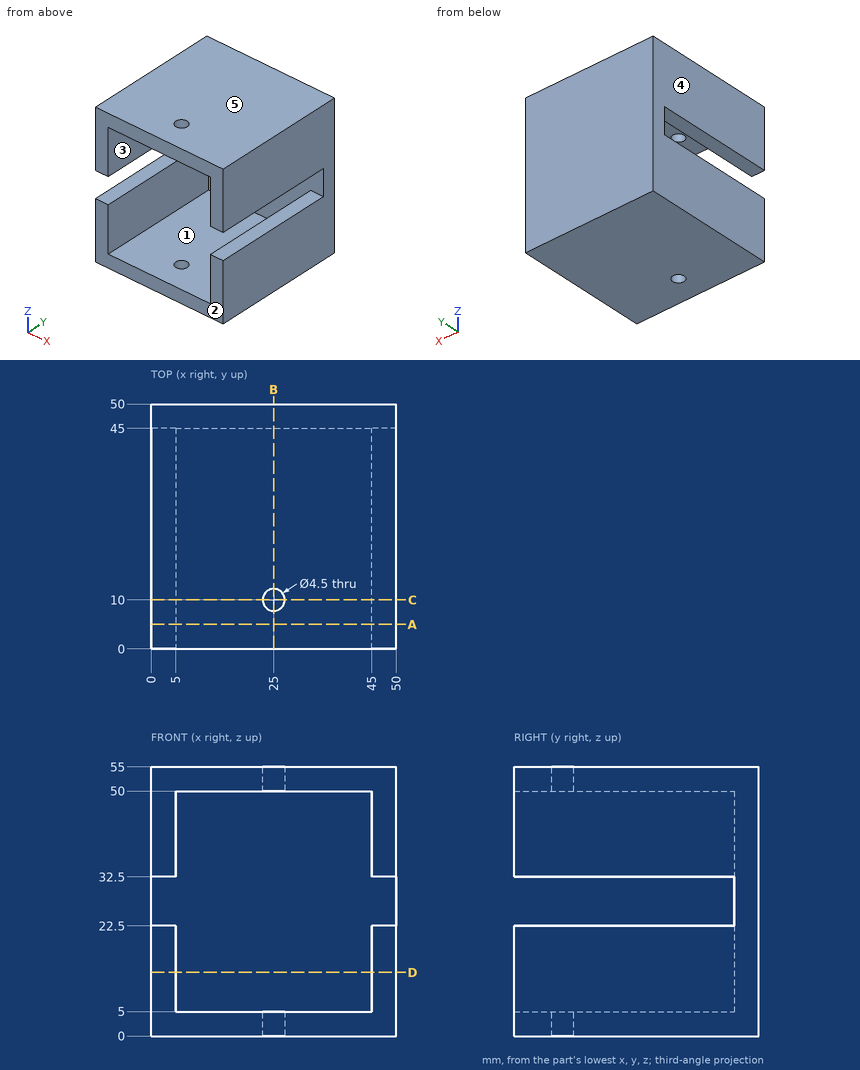
Can you work these out from the drawing? Everything is in mm from the part's minimum corner. A direction names the side the tool comes from. Coordinates: 2 decimals unless noted, no trailing zeros. Write each loop counter-clockwise with the first axis right and the second up, starting at its lowest first coordinate (ties: lowest second). Pieces come first, ordered by that corner, then holes. Notation, with made-up numbers: (-28.75, 40) -> (27.25, 40) arc R22 cw to (27.25, 53) -> close; hole circle Ø4 at (-14.75, 63). An arc over 180 degrees is marked (long way). Write each question's results on one line, items separated by ' | '. Start each with the question number.
Q1. Imagine slicing it at B-B (x = 25). Write out the boundary of the cut face in (y, z).
Q2. On a 3-axis mill with a long thin cutter (end or side, diameter ignored), from which of +Z, -Z, +X, -X, +Y, -Y can I reach the whole of each face in a straight line? I mean the marked faces 1 and 2. Say none if no direction works.
Q3. Imagine slicing it at D-D (z = 13). Write out the boundary of the cut face in (x, y).
Q4. If I drill on probe 1 along Z at (x, y) = (9, 38.5); probe 2 along Z at (x, y) = (3, 36); probe 3 along X at (y, z) = (15, 44), over which ranges is the centre line in solid material (lowest first)?
Q5. Imagine slicing it at A-A (y = 5). Write out the boundary of the cut face in (x, z).
Q6. We'd pull the mould along X, two halves only. Please class the marked faces 3, 4 and 5: +X half, -X half, draft (parallel to the pull), parting line (faces both ways), or undercut.
Q7. Imagine slicing it at C-C (y = 10). Write out the boundary of the cut face in (x, z), then the cut area to 3 significant figures.
Taken from the geometry:
1) outline: (0, 0) -> (7.75, 0) -> (7.75, 5) -> (0, 5) -> close; (0, 50) -> (7.75, 50) -> (7.75, 55) -> (0, 55) -> close; (12.25, 0) -> (50, 0) -> (50, 55) -> (12.25, 55) -> (12.25, 50) -> (45, 50) -> (45, 5) -> (12.25, 5) -> close
2) face 1: -Y | face 2: +Z, -Z, +X, -X, -Y
3) outline: (0, 0) -> (5, 0) -> (5, 45) -> (45, 45) -> (45, 0) -> (50, 0) -> (50, 50) -> (0, 50) -> close
4) probe 1: z = 0 to 5, 50 to 55 | probe 2: z = 0 to 22.5, 32.5 to 55 | probe 3: x = 0 to 5, 45 to 50
5) outline: (0, 0) -> (50, 0) -> (50, 22.5) -> (45, 22.5) -> (45, 5) -> (5, 5) -> (5, 22.5) -> (0, 22.5) -> close; (0, 32.5) -> (5, 32.5) -> (5, 50) -> (45, 50) -> (45, 32.5) -> (50, 32.5) -> (50, 55) -> (0, 55) -> close
6) face 3: undercut | face 4: -X half | face 5: draft
7) outline: (0, 0) -> (22.75, 0) -> (22.75, 5) -> (5, 5) -> (5, 22.5) -> (0, 22.5) -> close; (0, 32.5) -> (5, 32.5) -> (5, 50) -> (22.75, 50) -> (22.75, 55) -> (0, 55) -> close; (27.25, 0) -> (50, 0) -> (50, 22.5) -> (45, 22.5) -> (45, 5) -> (27.25, 5) -> close; (27.25, 50) -> (45, 50) -> (45, 32.5) -> (50, 32.5) -> (50, 55) -> (27.25, 55) -> close | area: 805 mm^2
